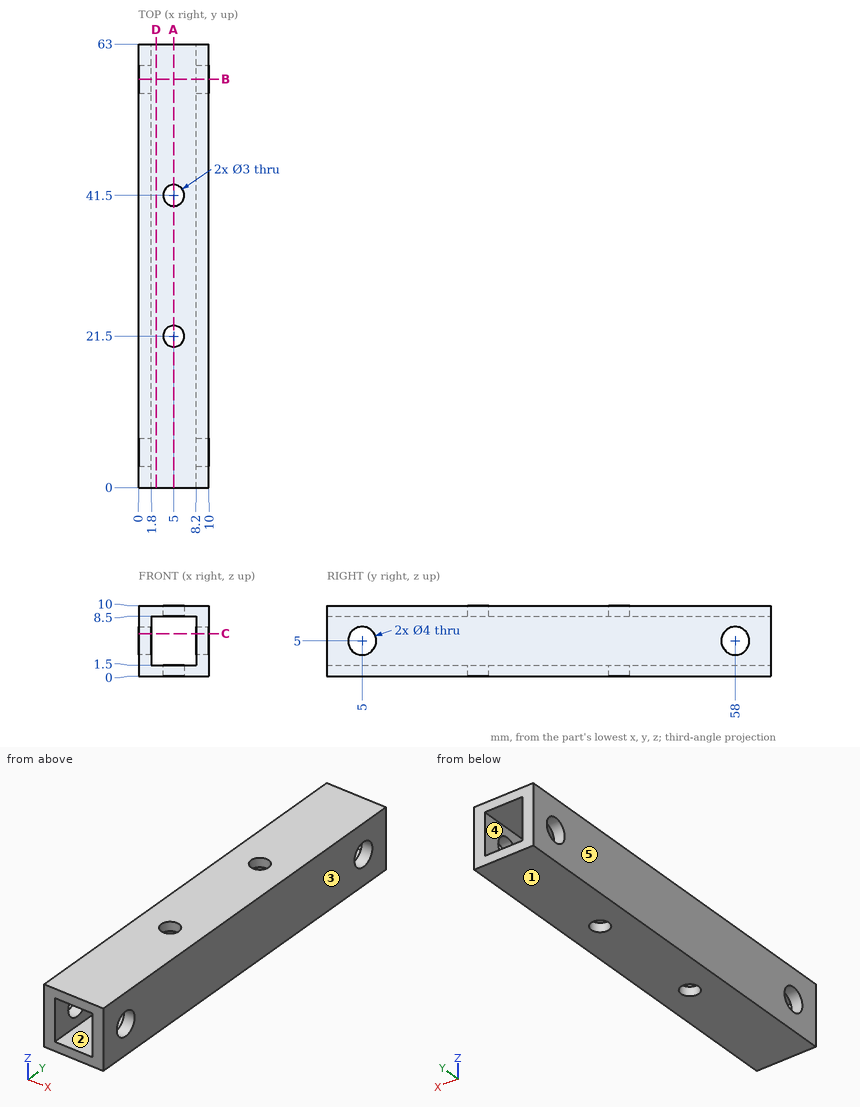
Input: dimensioned drawing with shaded views. Units: mm. Origin: part minimum x, y, z. A direction names the side the tool comes from. Coordinates: 2 decimals unless noted, no trailing zeros. Order: outer loops, then holes, each group sorted by start corner. A loop starts at its lowest first (then second) coordinate and runs counter-clockwise, first axis right, second up.
1. Cut plane A-A, the plane x = 5. Return loops of the section in (y, z), plus the area to 3 significant figures.
Checked values:
outline: (0, 0) - (20, 0) - (20, 1.5) - (0, 1.5) - close; (0, 8.5) - (20, 8.5) - (20, 10) - (0, 10) - close; (23, 0) - (40, 0) - (40, 1.5) - (23, 1.5) - close; (23, 8.5) - (40, 8.5) - (40, 10) - (23, 10) - close; (43, 0) - (63, 0) - (63, 1.5) - (43, 1.5) - close; (43, 8.5) - (63, 8.5) - (63, 10) - (43, 10) - close
area: 171 mm2
2. Contact query for a flat-ended pin moving along its axis: P1, Ø3.5, axis at x = 5, y = 21.5, coming from the +Z side. Output: stop coordinate, or through.
Checked values:
P1: stops at z = 10
3. Draft query along X for the marked faces 1, 2 and 3. Return one class per face: +X half, -X half, draft (parallel to the pull), parting line (faces both ways), or undercut.
Checked values:
face 1: draft
face 2: undercut
face 3: +X half
4. Cut plane C-C, the plane z = 6. Return loops of the section in (x, y), plus the area to 3 significant figures.
Checked values:
outline: (0, 0) - (1.8, 0) - (1.8, 3.27) - (0, 3.27) - close; (0, 6.73) - (1.8, 6.73) - (1.8, 56.27) - (0, 56.27) - close; (0, 59.73) - (1.8, 59.73) - (1.8, 63) - (0, 63) - close; (8.2, 0) - (10, 0) - (10, 3.27) - (8.2, 3.27) - close; (8.2, 6.73) - (10, 6.73) - (10, 56.27) - (8.2, 56.27) - close; (8.2, 59.73) - (10, 59.73) - (10, 63) - (8.2, 63) - close
area: 202 mm2
5. Cut plane D-D, the plane x = 2.5. Return loops of the section in (y, z), plus the area to 3 significant figures.
Checked values:
outline: (0, 0) - (63, 0) - (63, 1.5) - (0, 1.5) - close; (0, 8.5) - (63, 8.5) - (63, 10) - (0, 10) - close
area: 189 mm2
6. Cut plane B-B, the plane y = 58. Return loops of the section in (x, z).
Checked values:
outline: (0, 0) - (10, 0) - (10, 3) - (8.2, 3) - (8.2, 1.5) - (1.8, 1.5) - (1.8, 3) - (0, 3) - close; (0, 7) - (1.8, 7) - (1.8, 8.5) - (8.2, 8.5) - (8.2, 7) - (10, 7) - (10, 10) - (0, 10) - close
7. Access query for the marked faces 4 and 5. Directions: +Z, -Z, +X, -X, +Y, -Y. A direction counts if a zero-diameter tool reaches every point of the face in a straight line with its end or side. Return the directions, or none.
Checked values:
face 4: +Y, -Y
face 5: +Z, -Z, -X, +Y, -Y
8. Ray query, line 1 along Y through (x, z) = (1.05, 5); line 2 along Y through (x, z) = (5, 9.5); line 3 along Z through (x, y) = (7.75, 6.5). Return the intervals inside material, ascending.
Checked values:
line 1: y = 0 to 3, 7 to 56, 60 to 63
line 2: y = 0 to 20, 23 to 40, 43 to 63
line 3: z = 0 to 1.5, 8.5 to 10
